Model file for the job. Use its own axes, mm. A direction names the side the tool comes from. Round coordinates to 2 decimals unless told otherwise and drop trailing zeros. Order: outer loops, then holes, each group sorted by start corner. A loop starts at its lowest first (then second) coordinate and runs counter-clockwise, first axis right, second up. Notation, with made-up numbers: (-10, -30.75) -> (48, -30.75) arc R15 cw to (48, -21.75) -> close; hole circle Ø10 at (54.25, 0). An arc over 180 degrees is marked (long way). Use CSV: the item, a comma, the result in double quotes.
```python
from build123d import *

# Parameters (mm, degrees)
F1_DEPTH    = 76.2
F2_R        = 12.7
F3_DEPTH    = 38.1
F5_DEPTH    = 25.4
F6_T1_DEPTH = 215.9
F7_R        = 38.1
F8_R        = 19.05
F8_R_2      = 12.7
F9_DEPTH    = 6.35


# Not quite as in the source:
# - a fillet or chamfer that OpenCascade refuses, or shapes differently, is made with other operations: its cross-section is extruded or revolved along the edge and cut away or added


with BuildPart() as f1:
    # F0 (on Front) → F1 (new body, symmetric)
    with BuildSketch(Plane.XZ):
        Polygon((-76.2, 0), (0, 0), (0, 152.4), (-25.4, 152.4), (-25.4, 25.4), (-76.2, 25.4), align=None)
    extrude(amount=F1_DEPTH, both=True)

    # F2 (on face) → F3 (cut)
    with BuildSketch(Plane.YZ):
        with Locations((0, 114.3)):
            Circle(F2_R)
    extrude(amount=-F3_DEPTH, mode=Mode.SUBTRACT)

    # F4 (on face) → F5 (cut)
    with BuildSketch(Plane.XY.offset(25.4)):
        with BuildLine():
            Line((-63.5, 12.7), (-76.2, 12.7))
            Line((-76.2, 12.7), (-76.2, -12.7))
            Line((-76.2, -12.7), (-63.5, -12.7))
            ThreePointArc((-63.5, -12.7), (-50.8, 0), (-63.5, 12.7))
        make_face()
    extrude(amount=-F5_DEPTH, mode=Mode.SUBTRACT)

    # F6: fillet of radius 38.1 on 1 edges, made by hand

    # F6_s2 → F6_t1 (cut)
    with BuildSketch(Plane.YZ.offset(-120.65)):
        with BuildLine():
            add(Edge.make_bspline(
                [(-76.2, 114.3), (-76.2, 152.4), (-38.1, 152.4)],
                knots=[0, 0, 0, 1, 1, 1], degree=2, weights=[1, 1, 1]))
            Line((-38.1, 152.4), (-76.2, 152.4))
            Line((-76.2, 152.4), (-76.2, 114.3))
        make_face()
    extrude(amount=F6_T1_DEPTH, mode=Mode.SUBTRACT)

    # F7
    f7_edges = [f1.edges().sort_by_distance(p)[0] for p in [
        (-12.7, 76.2, 152.4),
    ]]
    fillet(f7_edges, radius=F7_R)

    # F8 (on face) → F9 (cut)
    with BuildSketch(Plane(origin=(-25.4, 0, 0), x_dir=(0, -1, 0), z_dir=(-1, 0, 0))):
        with Locations((0, 114.3)):
            Circle(F8_R)
        with Locations((0, 114.3)):
            Circle(F8_R_2, mode=Mode.SUBTRACT)
    extrude(amount=-F9_DEPTH, mode=Mode.SUBTRACT)


solid = f1.part
```
Q1. Probe line 1 along Z through (x, y) = (-22.75, 0); line 2 along Y through (x, z) = (-8, 114); line 3 along Y through (x, z) = (-21, 114). List the from-to ranges inside material, lowest first.
From the geometry:
line 1,"z = 0 to 95.25, 133.35 to 152.4"
line 2,"y = -76.2 to -12.7, 12.7 to 76.2"
line 3,"y = -76.2 to -19.05, 19.05 to 76.2"
Q2. Which spindle directions (+Z, -Z, +X, -X, +Y, -Y) get a long thin tool onto all of the face, cutting with end or side? Do faces 5 (the flat face through (0, -1, 75)), 6 (the flat face through (-70, 12.7, 13)), 7 (the flat face through (-25.4, -1, 90)). Say none if no direction does.
From the geometry:
face 5,"+Z, -Z, +X, +Y, -Y"
face 6,"+Z, -Z, -X"
face 7,"+Z, -X, +Y, -Y"
Q3. Cut at D-D (x = -32.5). Give the cut face in (y, z), plus the area to 3 significant figures.
From the geometry:
outline,"(-76.2, 0) -> (76.2, 0) -> (76.2, 25.4) -> (-76.2, 25.4) -> close"
area,"3,870 mm²"
Q4. Pin check, flat tips, straight feed: pin 1 (10 mm diameter, centred on y = -50.5, z = 51, fed in from -X); pin 2 (5 mm diameter, centred on x = -31, y = -13, fed in from -Z); pin 3 (1.5 mm diameter, centred on x = -63, y = 34.5, fed in from +Z). Stop position of each tip, or through.
From the geometry:
pin 1,"stops at x = -25.4"
pin 2,"stops at z = 0"
pin 3,"stops at z = 25.4"
Q5. Cut at B-B (y = 28.5). Give the cut face in (x, z).
From the geometry:
outline,"(-76.2, 0) -> (0, 0) -> (0, 152.4) -> (-25.4, 152.4) -> (-25.4, 25.4) -> (-76.2, 25.4) -> close"
Q6. Mould opens along Z. For faces 1 (the cylindrical face through (-22.269, 4.13, 95.703)), 2 (the flat face through (-19.05, -4, 102)), 3 (the flat face through (-76.2, -45, 13)), 4 (the flat face through (-39, -1, 0)) say: +Z half, -Z half, draft (parallel to the pull), parting line (faces both ways), or undercut.
From the geometry:
face 1,"undercut"
face 2,"undercut"
face 3,"draft"
face 4,"-Z half"
Q7. Cut at A-A (y = 0). Give the cut face in (x, z), plus the area to 3 significant figures.
From the geometry:
outline,"(-50.8, 0) -> (0, 0) -> (0, 101.6) -> (-19.05, 101.6) -> (-19.05, 95.25) -> (-25.4, 95.25) -> (-25.4, 25.4) -> (-50.8, 25.4) -> close; (-25.4, 133.35) -> (-19.05, 133.35) -> (-19.05, 127) -> (0, 127) -> (0, 152.4) -> (-25.4, 152.4) -> close"
area,"3,790 mm²"
Q8. Cut at C-C (z = 85). Give the cut face in (x, y).
From the geometry:
outline,"(-25.4, -76.2) -> (0, -76.2) -> (0, 76.2) -> (-25.4, 76.2) -> close"
